Work out the finished part from the listing and answer in its coordinate system (mm). Face numbers are marked on the shaded views. A direction names the side the tool comes from. Give positions to 0.01 mm unless a question says otherwise; leave off trailing zeros. Loops run counter-clockwise (first coordinate to the right, second up) from the corner with the lowest first, then second, coordinate; pieces in that order, holes last. Notation, with made-up numbers: (-23.5, 26) -> (20.5, 26) arc R19 cw to (20.5, 48) -> close; hole circle Ø1 at (0, 48). An arc over 180 degrees is marked (long way). Answer as CSV lines item,"result". Start each with the question number.
1. Find section C-C, the plane x = 6.5. Give the vertices of the cut face in (y, z).
2. Find section D-D, the plane z = -9.75. Give the vertices of the cut face in (x, y), and give its area (3 significant figures).
3. A tool of negligible diameter and unlimited length cuts with its end or side. For the marked faces 4, 5, 6, 7 and 8, from which of +Z, -Z, +X, -X, +Y, -Y can it reach the whole face along a straight path? Write none if from no direction.
4. Find the intervals of material crossed by line 1 along X through (y, z) = (2.25, 0); line 2 along Z through (x, y) = (9, 1); line 3 along Z through (x, y) = (-9, 2.5), in increasing order.
5. Find section B-B, the plane x = 0. Give the vertices of the cut face in (y, z), and give its area (3 significant figures).
6. Determine the mould class of the marked faces 1, 2 and 3 for opening direction X: +X half, -X half, draft (parallel to the pull), parting line (faces both ways), or undercut.
7. Flat-ended cylindrical pins translate along their axes: pin 1 Ø4 at (x, z) = (0.5, -0.5) entering from +Y; pin 2 Ø1.5 at (y, z) = (4.5, 6.5) entering from -X. Find the tip coordinate at first contact, or state that the pin passes through.
8. Find section A-A, the plane z = 0. Give the vertices of the cut face in (x, y), and give its area (3 significant figures).
from build123d import *

# Parameters (mm, degrees)
SKETCH1_R           = 8.509
BOSS_EXTRUDE1_DEPTH = 7.55
SKETCH2_R           = 1.5875
CUT_EXTRUDE1_DEPTH  = 15.205937561
BOSS_EXTRUDE2_DEPTH = 7.55
CIRPATTERN1_COUNT   = 6


with BuildPart() as part:
    # Sketch1 → Boss-Extrude1 (new body)
    with BuildSketch(Plane(origin=(0, 0, 0), x_dir=(1, 0, 0), z_dir=(0, 1, 0))):
        with Locations(Location((0, 0, 0), (0, 0, 270))):
            Circle(SKETCH1_R)
    extrude(amount=BOSS_EXTRUDE1_DEPTH)

    # Sketch2 → Cut-Extrude1 (cut, through all)
    with BuildSketch(Plane(origin=(0, 7.55, 0), x_dir=(1, 0, 0), z_dir=(0, 1, 0))):
        with Locations(Location((0, 0, 0), (0, 0, 270))):
            Circle(SKETCH2_R)
    extrude(amount=-CUT_EXTRUDE1_DEPTH, mode=Mode.SUBTRACT)

    # Sketch3 → Boss-Extrude2 (add, through all)
    with BuildSketch(Plane(origin=(0, 7.55, 0), x_dir=(1, 0, 0), z_dir=(0, 1, 0))):
        with BuildLine():
            Line((-1.082882935, 12.042261501), (1.725110007, 11.967150578))
            ThreePointArc((1.725110007, 11.967150578), (2.393433601, 11.686456973), (2.69653959, 11.027995064))
            Line((2.69653959, 11.027995064), (2.879609723, 8.006930051))
            ThreePointArc((2.879609723, 8.006930051), (0.227525612, 8.505957506), (-2.447443894, 8.149423255))
            Line((-2.447443894, 8.149423255), (-2.103130346, 11.156381297))
            ThreePointArc((-2.103130346, 11.156381297), (-1.765256626, 11.797697659), (-1.082882935, 12.042261501))
        make_face()
    boss_extrude2 = extrude(amount=-BOSS_EXTRUDE2_DEPTH)

    # CirPattern1: Boss-Extrude2 ×6 about axis
    cirpattern1_axis = Axis((0, 0, 0), (0, 1, 0))
    for i in range(1, CIRPATTERN1_COUNT):
        add(boss_extrude2.rotate(cirpattern1_axis, i * 360 / CIRPATTERN1_COUNT))


solid = part.part
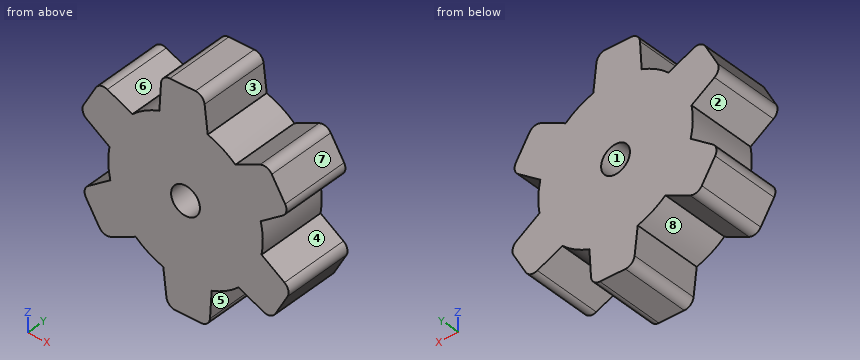
Resolved:
1,outline,"(0, -6.48) -> (7.55, -6.48) -> (7.55, 7) -> (0, 7) -> close"
2,outline,"(-2.26, 0) -> (2.77, 0) -> (2.77, 7.55) -> (-2.26, 7.55) -> close"
2,area,"38.0 mm^2"
3,face 4,"+X, +Y, -Y"
3,face 5,"-Z, +X, +Y, -Y"
3,face 6,"+Z, +Y, -Y"
3,face 7,"+Z, +X, +Y, -Y"
3,face 8,"-Z, +Y, -Y"
4,line 1,"x = -8.51 to -1.59, 1.59 to 8.51"
4,line 2,"z = -7.48 to -1.92, 2.49 to 7.89"
4,line 3,"z = -7.89 to -2.49, 1.92 to 7.48"
5,outline,"(0, -12.01) -> (7.55, -12.01) -> (7.55, -1.59) -> (0, -1.59) -> close; (0, 1.59) -> (7.55, 1.59) -> (7.55, 12.01) -> (0, 12.01) -> close"
5,area,"157 mm^2"
6,face 1,"undercut"
6,face 2,"-X half"
6,face 3,"+X half"
7,pin 1,"stops at y = 7.55"
7,pin 2,"stops at x = -10.54"
8,outline,"(-8.51, 0) -> (-1.59, 0) -> (-1.59, 7.55) -> (-8.51, 7.55) -> close; (1.59, 0) -> (8.51, 0) -> (8.51, 7.55) -> (1.59, 7.55) -> close"
8,area,"105 mm^2"
